The listing builds one solid part. Answer for the finished solid, in the listing's coordinates (mm). Coordinates: 2 decimals unless noted, no trailing zeros. Loops run counter-clockwise (first coordinate to the right, second up) from the corner with the lowest first, then second, coordinate; pieces in that order, holes last. Notation, with made-up numbers: M 17.25,-37 L 31.25,-37 A16 ccw 31.25,-25 Z; hole C 23.5,49 d9. An arc over 180 degrees is marked long. Answer as a JSON object with one key per item and string values. Group by question number.
1. A cutting plane is placed at B-B on z = 1.2. Give the vertices of the cut face in (x, y), and give its area (3 significant figures).
2. A cutting plane is placed at D-D on y = 3. Give the vertices of the cut face in (x, z).
3. Given pin 1 (2 mm diameter, centred on y = -2.5, z = 1, fed in from +X), flat-ended and moving along its own axis, determine where the tip first touches the part or whether it passes through.
4. A cutting plane is placed at A-A on y = 0. Give the vertices of the cut face in (x, z).
5. Straight lines are drawn through the part: L1, parallel to Y at x = 21, z = 3.3; L2, parallel to X at y = -1, z = 2.65; L3, parallel to X at y = -1.25, z = 3.1. For each, find the intervals that lie inside material, in ascending order.
6. A cutting plane is placed at C-C on x = -1.5. Give the vertices of the cut face in (y, z), and give its area (3 significant figures).
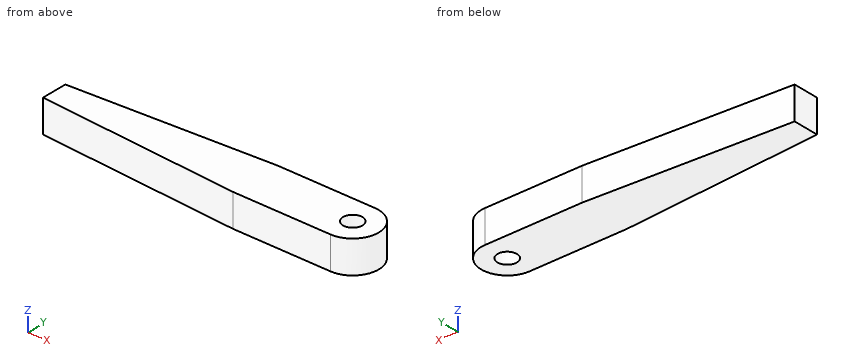
from build123d import *

# Parameters (mm, degrees)
ESQUISSE1_R        = 1.5
BOSS_EXTRU_1_DEPTH = 5


with BuildPart() as part:
    # Esquisse1 → Boss.-Extru.1 (new body)
    with BuildSketch(Plane.XY):
        with BuildLine():
            Line((6, 4), (21, 4))
            ThreePointArc((21, 4), (25, 0), (21, -4))
            Line((21, -4), (6, -4))
            Line((6, -4), (-25, -2))
            Line((-25, -2), (-25, 2))
            Line((-25, 2), (6, 4))
        make_face()
        with Locations((21, 0)):
            Circle(ESQUISSE1_R, mode=Mode.SUBTRACT)
    extrude(amount=BOSS_EXTRU_1_DEPTH)


solid = part.part
From the geometry:
{
 "1": {"outline": "M -25,-2 L 6,-4 L 21,-4 A4 ccw 21,4 L 6,4 L -25,2 Z; hole C 21,0 d3", "area": "324 mm²"},
 "2": {"outline": "M -9.5,0 L 23.65,0 L 23.65,5 L -9.5,5 Z"},
 "3": {"pin 1": "stops at x = 24.71"},
 "4": {"outline": "M -25,0 L 19.5,0 L 19.5,5 L -25,5 Z; M 22.5,0 L 25,0 L 25,5 L 22.5,5 Z"},
 "5": {"L1": "y = -4 to -1.5, 1.5 to 4", "L2": "x = -25 to 19.88, 22.12 to 24.87", "L3": "x = -25 to 20.17, 21.83 to 24.8"},
 "6": {"outline": "M -3.52,0 L 3.52,0 L 3.52,5 L -3.52,5 Z", "area": "35.2 mm²"}
}
